For this review, take the finished solid that the model builds, in its own axes (mm). Face numbers are marked on the shaded views. A direction names the side the tool comes from. Coordinates: 2 decimals unless noted, no trailing zeros. Write each loop counter-clockwise with the first axis right and the second up, starting at its lowest first coordinate (ties: lowest second). Pieces come first, ordered by that corner, then holes. Notation, with made-up numbers: M -14.5,2 L -7.5,2 A16 cw -7.5,33 Z; hole C 27,13.5 d1. An arc over 180 degrees is marked long. One line per question, with ' | ' between items.
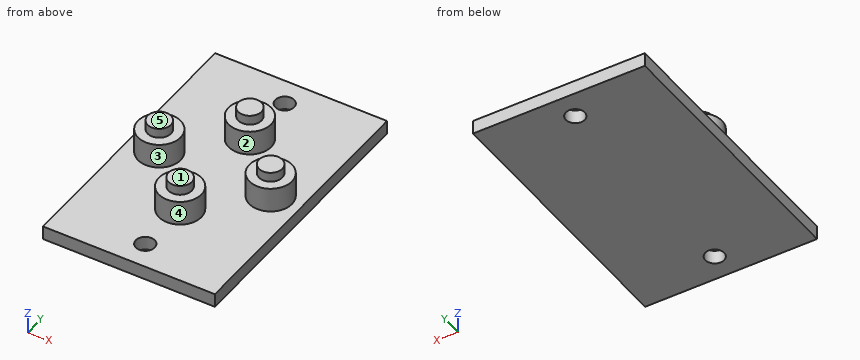
from build123d import *

# Parameters (mm, degrees)
SKETCH1_W           = 25
SKETCH1_H           = 40
BOSS_EXTRUDE1_DEPTH = 2
SKETCH2_R           = 3.1
BOSS_EXTRUDE2_DEPTH = 3.6
SKETCH3_R           = 1.7
BOSS_EXTRUDE3_DEPTH = 1.4
SKETCH4_R           = 1.7
BOSS_EXTRUDE4_DEPTH = 1.4
SKETCH5_R           = 1.7
BOSS_EXTRUDE5_DEPTH = 1.4
SKETCH6_R           = 1.7
BOSS_EXTRUDE6_DEPTH = 1.4
SKETCH7_R           = 1.375
CUT_EXTRUDE1_DEPTH  = 3


with BuildPart() as part:
    # Sketch1 → Boss-Extrude1 (new body)
    with BuildSketch(Plane.XY):
        Rectangle(SKETCH1_W, SKETCH1_H)
    extrude(amount=BOSS_EXTRUDE1_DEPTH)

    # Sketch2 → Boss-Extrude2 (add)
    with BuildSketch(Plane.XY.offset(2)):
        with Locations((-8.1, 0)):
            Circle(SKETCH2_R)
        with Locations((8.1, 0)):
            Circle(SKETCH2_R)
        with Locations((0, 8.1)):
            Circle(SKETCH2_R)
        with Locations((0, -8.1)):
            Circle(SKETCH2_R)
    extrude(amount=BOSS_EXTRUDE2_DEPTH)

    # Sketch3 → Boss-Extrude3 (add)
    with BuildSketch(Plane.XY.offset(5.6)):
        with Locations((0, 8.1)):
            Circle(SKETCH3_R)
    extrude(amount=BOSS_EXTRUDE3_DEPTH)

    # Sketch4 → Boss-Extrude4 (add)
    with BuildSketch(Plane.XY.offset(5.6)):
        with Locations((-8.1, 0)):
            Circle(SKETCH4_R)
    extrude(amount=BOSS_EXTRUDE4_DEPTH)

    # Sketch5 → Boss-Extrude5 (add)
    with BuildSketch(Plane.XY.offset(5.6)):
        with Locations((8.1, 0)):
            Circle(SKETCH5_R)
    extrude(amount=BOSS_EXTRUDE5_DEPTH)

    # Sketch6 → Boss-Extrude6 (add)
    with BuildSketch(Plane.XY.offset(5.6)):
        with Locations((0, -8.1)):
            Circle(SKETCH6_R)
    extrude(amount=BOSS_EXTRUDE6_DEPTH)

    # Sketch7 → Cut-Extrude1 (cut)
    with BuildSketch(Plane.XY.offset(2)):
        with Locations((0, 16.2)):
            Circle(SKETCH7_R)
        with Locations((0, -16.2)):
            Circle(SKETCH7_R)
    extrude(amount=-CUT_EXTRUDE1_DEPTH, mode=Mode.SUBTRACT)


solid = part.part
1) We need section D-D on z = 3.5. State the section outline as (x, y) points.
Responses:
outline: C -8.1,0 d6.2; C 0,-8.1 d6.2; C 0,8.1 d6.2; C 8.1,0 d6.2
2) We need section B-B on y = 16.2. State the section outline as (x, z) points (3 decimals), then the cut area to 3 significant figures.
Responses:
outline: M -12.5,0 L -1.375,0 L -1.375,2 L -12.5,2 Z; M 1.375,0 L 12.5,0 L 12.5,2 L 1.375,2 Z | area: 44.5 mm^2
3) The part is to be moulded in two halves that separate along Y. For the marked faces 3, 4 and 5, say which applies: +Y half, -Y half, draft (parallel to the pull), parting line (faces both ways), or undercut.
Responses:
face 3: parting line | face 4: undercut | face 5: draft
4) We need section C-C on y = 8.1. State the section outline as (x, z) points.
Responses:
outline: M -12.5,0 L 12.5,0 L 12.5,2 L 3.1,2 L 3.1,5.6 L 1.7,5.6 L 1.7,7 L -1.7,7 L -1.7,5.6 L -3.1,5.6 L -3.1,2 L -12.5,2 Z
5) Machinability: for the marked faces 1 and 2, which of the approach directions +Z, -Z, +X, -X, +Y, -Y give a long, thin tool a straight path to every point of the face, cutting with its end or side? Answer none if there is none.
Responses:
face 1: +Z, +X, -X, +Y, -Y | face 2: +Z
6) Insertion check: pin 1 Ø1.6 at (x, y) = (0, -16.2) entering from +Z; pin 2 Ø2 at (x, z) = (0, 6) entering from +Y; pin 3 Ø1.5 at (x, z) = (2.5, 5) entering from -Y; pin 4 Ø7.5 at (x, y) = (2.5, 0) entering from +Z. Each pin has a flat end and moves straight along its axis. Give the tip position at first contact, or say it passes through.
Responses:
pin 1: through | pin 2: y = 11.2 | pin 3: y = -10.66 | pin 4: z = 5.6
7) To check wall thickness, follow line 1 along Y through (x, z) = (0, 1.4) (3 decimals); line 2 along Z through (x, y) = (-0.5, 1.5); line 3 along X through (y, z) = (2, 5). State the ranges of each line that lie inside material, in increasing order. Write a range as [from, to].
Responses:
line 1: [-20, -17.575], [-14.825, 14.825], [17.575, 20] | line 2: [0, 2] | line 3: [-10.47, -5.73], [5.73, 10.47]
8) We need section A-A on x = 0. State the section outline as (y, z) points (3 decimals), then the cut area to 3 significant figures.
Responses:
outline: M -20,0 L -17.575,0 L -17.575,2 L -20,2 Z; M -14.825,0 L 14.825,0 L 14.825,2 L 11.2,2 L 11.2,5.6 L 9.8,5.6 L 9.8,7 L 6.4,7 L 6.4,5.6 L 5,5.6 L 5,2 L -5,2 L -5,5.6 L -6.4,5.6 L -6.4,7 L -9.8,7 L -9.8,5.6 L -11.2,5.6 L -11.2,2 L -14.825,2 Z; M 17.575,0 L 20,0 L 20,2 L 17.575,2 Z | area: 123 mm^2
